Part model, mm, in its own coordinate system. Face numbers are marked on the shaded views. Give positions to 0.01 mm unless a question says otherwise; leave off trailing zeros. Order: outer loops, then holes, each group sorted by start corner. A loop starts at its lowest first (then second) coordinate and runs counter-clockwise, first axis right, second up. Notation, with made-up numbers: (69, -35.75) - (120, -35.75) arc R24 cw to (120, -15.75) - close; hole circle Ø3 at (67, 42.5). An arc over 180 degrees is marked (long way). One line per item, written item: value.
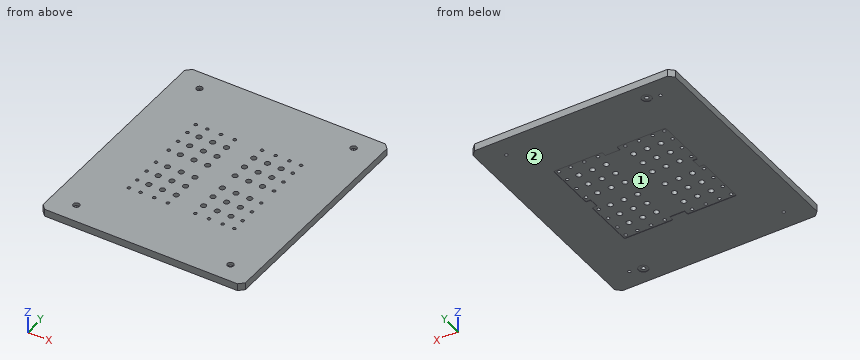
```python
from build123d import *

# Parameters (mm, degrees)
F0_W           = 210
F0_H           = 240
F1_DEPTH       = 7.5
F3_D           = 3.15
F3_CBORE_D     = 6.5
F3_CBORE_DEPTH = 3
F5_D           = 4.2
F5_DEPTH       = 5.5
F5_CBORE_D     = 10
F5_CBORE_DEPTH = 0.5
F5_TIP         = 1.2618073
F7_D           = 5.5
F9_D           = 3.3
F10_R          = 1.65
F10_R_2        = 2.75
F11_DEPTH      = 0.5
F12_SIZE       = 5
F13_R          = 1.5


with BuildPart() as f1:
    # F0 (on Top) → F1 (new body)
    with BuildSketch(Plane.XY):
        Rectangle(F0_W, F0_H)
    extrude(amount=F1_DEPTH)

    # F3 (through all)
    with Locations(Plane.XY.offset(7.5)):
        with Locations((-80, 100), (80, 100), (-80, -100), (80, -100)):
            CounterBoreHole(F3_D / 2, F3_CBORE_D / 2, F3_CBORE_DEPTH)

    # F5
    with Locations(Plane(origin=(0, 0, 0), x_dir=(1, 0, 0), z_dir=(0, 0, -1))):
        with Locations((-67.5, -103), (67.5, 103)):
            CounterBoreHole(F5_D / 2, F5_CBORE_D / 2, F5_CBORE_DEPTH, depth=F5_DEPTH)
            with Locations((0, 0, -(F5_DEPTH + F5_TIP / 2))):  # 118° drill point
                Cone(0, F5_D / 2, F5_TIP, mode=Mode.SUBTRACT)

    # F7 (through all)
    with Locations(Plane.XY.offset(7.5)):
        with Locations((-42.6, 40.75), (-28.4, 40.75), (-14.2, 40.75), (14.2, 40.75), (28.4, 40.75), (42.6, 40.75), (-42.6, 25.55), (-28.4, 25.55), (-14.2, 25.55), (14.2, 25.55), (28.4, 25.55), (42.6, 25.55), (42.6, 10.35), (28.4, 10.35), (14.2, 10.35), (-14.2, 10.35), (-28.4, 10.35), (-42.6, 10.35), (-42.6, -10.35), (-28.4, -10.35), (-14.2, -10.35), (14.2, -10.35), (28.4, -10.35), (42.6, -10.35), (42.6, -25.55), (28.4, -25.55), (14.2, -25.55), (-14.2, -25.55), (-28.4, -25.55), (-42.6, -25.55), (-42.6, -40.75), (-28.4, -40.75), (-14.2, -40.75), (14.2, -40.75), (28.4, -40.75), (42.6, -40.75)):
            Hole(F7_D / 2)

    # F9 (through all)
    with Locations(Plane.XY.offset(7.5)):
        with Locations((-54.65, 54.2), (-42.6, 54.2), (-28.4, 54.2), (-14.2, 54.2), (14.2, 54.2), (28.4, 54.2), (42.6, 54.2), (54.65, 54.2), (54.65, 40.75), (54.65, 25.55), (54.65, 10.35), (54.65, -10.35), (54.65, -25.55), (54.65, -40.75), (54.65, -54.2), (42.6, -54.2), (28.4, -54.2), (14.2, -54.2), (-14.2, -54.2), (-28.4, -54.2), (-42.6, -54.2), (-54.65, -54.2), (-54.65, -40.75), (-54.65, -25.55), (-54.65, -10.35), (-54.65, 10.35), (-54.65, 25.55), (-54.65, 40.75)):
            Hole(F9_D / 2)

    # F10 (on face) → F11 (cut)
    with BuildSketch(Plane(origin=(0, 0, 0), x_dir=(1, 0, 0), z_dir=(0, 0, -1))):
        with BuildLine():
            Line((7.5, -57.7), (56.625, -57.7))
            ThreePointArc((56.625, -57.7), (57.6856601718, -57.2606601718), (58.125, -56.2))
            Line((58.125, -56.2), (58.125, -5))
            Line((58.125, -5), (53.125, -5))
            Line((53.125, -5), (53.125, 5))
            Line((53.125, 5), (58.125, 5))
            Line((58.125, 5), (58.125, 56.2))
            ThreePointArc((58.125, 56.2), (57.6856601718, 57.2606601718), (56.625, 57.7))
            Line((56.625, 57.7), (7.5, 57.7))
            Line((7.5, 57.7), (7.5, 52.7))
            Line((7.5, 52.7), (-7.5, 52.7))
            Line((-7.5, 52.7), (-7.5, 57.7))
            Line((-7.5, 57.7), (-56.625, 57.7))
            ThreePointArc((-56.625, 57.7), (-57.6856601718, 57.2606601718), (-58.125, 56.2))
            Line((-58.125, 56.2), (-58.125, 5))
            Line((-58.125, 5), (-53.125, 5))
            Line((-53.125, 5), (-53.125, -5))
            Line((-53.125, -5), (-58.125, -5))
            Line((-58.125, -5), (-58.125, -56.2))
            ThreePointArc((-58.125, -56.2), (-57.6856601718, -57.2606601718), (-56.625, -57.7))
            Line((-56.625, -57.7), (-7.5, -57.7))
            Line((-7.5, -57.7), (-7.5, -52.7))
            Line((-7.5, -52.7), (7.5, -52.7))
            Line((7.5, -52.7), (7.5, -57.7))
        make_face()
        with Locations((-54.65, -54.2)):
            Circle(F10_R, mode=Mode.SUBTRACT)
        with Locations((-54.65, -40.75)):
            Circle(F10_R, mode=Mode.SUBTRACT)
        with Locations((-54.65, -25.55)):
            Circle(F10_R, mode=Mode.SUBTRACT)
        with Locations((-54.65, -10.35)):
            Circle(F10_R, mode=Mode.SUBTRACT)
        with Locations((-42.6, -54.2)):
            Circle(F10_R, mode=Mode.SUBTRACT)
        with Locations((-28.4, -54.2)):
            Circle(F10_R, mode=Mode.SUBTRACT)
        with Locations((-42.6, -40.75)):
            Circle(F10_R_2, mode=Mode.SUBTRACT)
        with Locations((-28.4, -40.75)):
            Circle(F10_R_2, mode=Mode.SUBTRACT)
        with Locations((-14.2, -54.2)):
            Circle(F10_R, mode=Mode.SUBTRACT)
        with Locations((-14.2, -40.75)):
            Circle(F10_R_2, mode=Mode.SUBTRACT)
        with Locations((-42.6, -25.55)):
            Circle(F10_R_2, mode=Mode.SUBTRACT)
        with Locations((-28.4, -25.55)):
            Circle(F10_R_2, mode=Mode.SUBTRACT)
        with Locations((-42.6, -10.35)):
            Circle(F10_R_2, mode=Mode.SUBTRACT)
        with Locations((-28.4, -10.35)):
            Circle(F10_R_2, mode=Mode.SUBTRACT)
        with Locations((-14.2, -25.55)):
            Circle(F10_R_2, mode=Mode.SUBTRACT)
        with Locations((-14.2, -10.35)):
            Circle(F10_R_2, mode=Mode.SUBTRACT)
        with Locations((14.2, -54.2)):
            Circle(F10_R, mode=Mode.SUBTRACT)
        with Locations((14.2, -40.75)):
            Circle(F10_R_2, mode=Mode.SUBTRACT)
        with Locations((28.4, -54.2)):
            Circle(F10_R, mode=Mode.SUBTRACT)
        with Locations((42.6, -54.2)):
            Circle(F10_R, mode=Mode.SUBTRACT)
        with Locations((28.4, -40.75)):
            Circle(F10_R_2, mode=Mode.SUBTRACT)
        with Locations((42.6, -40.75)):
            Circle(F10_R_2, mode=Mode.SUBTRACT)
        with Locations((14.2, -25.55)):
            Circle(F10_R_2, mode=Mode.SUBTRACT)
        with Locations((14.2, -10.35)):
            Circle(F10_R_2, mode=Mode.SUBTRACT)
        with Locations((28.4, -25.55)):
            Circle(F10_R_2, mode=Mode.SUBTRACT)
        with Locations((42.6, -25.55)):
            Circle(F10_R_2, mode=Mode.SUBTRACT)
        with Locations((28.4, -10.35)):
            Circle(F10_R_2, mode=Mode.SUBTRACT)
        with Locations((42.6, -10.35)):
            Circle(F10_R_2, mode=Mode.SUBTRACT)
        with Locations((54.65, -54.2)):
            Circle(F10_R, mode=Mode.SUBTRACT)
        with Locations((54.65, -40.75)):
            Circle(F10_R, mode=Mode.SUBTRACT)
        with Locations((54.65, -25.55)):
            Circle(F10_R, mode=Mode.SUBTRACT)
        with Locations((54.65, -10.35)):
            Circle(F10_R, mode=Mode.SUBTRACT)
        with Locations((-54.65, 10.35)):
            Circle(F10_R, mode=Mode.SUBTRACT)
        with Locations((-54.65, 25.55)):
            Circle(F10_R, mode=Mode.SUBTRACT)
        with Locations((-54.65, 40.75)):
            Circle(F10_R, mode=Mode.SUBTRACT)
        with Locations((-54.65, 54.2)):
            Circle(F10_R, mode=Mode.SUBTRACT)
        with Locations((-42.6, 10.35)):
            Circle(F10_R_2, mode=Mode.SUBTRACT)
        with Locations((-28.4, 10.35)):
            Circle(F10_R_2, mode=Mode.SUBTRACT)
        with Locations((-42.6, 25.55)):
            Circle(F10_R_2, mode=Mode.SUBTRACT)
        with Locations((-28.4, 25.55)):
            Circle(F10_R_2, mode=Mode.SUBTRACT)
        with Locations((-14.2, 10.35)):
            Circle(F10_R_2, mode=Mode.SUBTRACT)
        with Locations((-14.2, 25.55)):
            Circle(F10_R_2, mode=Mode.SUBTRACT)
        with Locations((-42.6, 40.75)):
            Circle(F10_R_2, mode=Mode.SUBTRACT)
        with Locations((-28.4, 40.75)):
            Circle(F10_R_2, mode=Mode.SUBTRACT)
        with Locations((-42.6, 54.2)):
            Circle(F10_R, mode=Mode.SUBTRACT)
        with Locations((-28.4, 54.2)):
            Circle(F10_R, mode=Mode.SUBTRACT)
        with Locations((-14.2, 40.75)):
            Circle(F10_R_2, mode=Mode.SUBTRACT)
        with Locations((-14.2, 54.2)):
            Circle(F10_R, mode=Mode.SUBTRACT)
        with Locations((14.2, 10.35)):
            Circle(F10_R_2, mode=Mode.SUBTRACT)
        with Locations((14.2, 25.55)):
            Circle(F10_R_2, mode=Mode.SUBTRACT)
        with Locations((28.4, 10.35)):
            Circle(F10_R_2, mode=Mode.SUBTRACT)
        with Locations((42.6, 10.35)):
            Circle(F10_R_2, mode=Mode.SUBTRACT)
        with Locations((28.4, 25.55)):
            Circle(F10_R_2, mode=Mode.SUBTRACT)
        with Locations((42.6, 25.55)):
            Circle(F10_R_2, mode=Mode.SUBTRACT)
        with Locations((14.2, 40.75)):
            Circle(F10_R_2, mode=Mode.SUBTRACT)
        with Locations((14.2, 54.2)):
            Circle(F10_R, mode=Mode.SUBTRACT)
        with Locations((28.4, 40.75)):
            Circle(F10_R_2, mode=Mode.SUBTRACT)
        with Locations((42.6, 40.75)):
            Circle(F10_R_2, mode=Mode.SUBTRACT)
        with Locations((28.4, 54.2)):
            Circle(F10_R, mode=Mode.SUBTRACT)
        with Locations((42.6, 54.2)):
            Circle(F10_R, mode=Mode.SUBTRACT)
        with Locations((54.65, 10.35)):
            Circle(F10_R, mode=Mode.SUBTRACT)
        with Locations((54.65, 25.55)):
            Circle(F10_R, mode=Mode.SUBTRACT)
        with Locations((54.65, 40.75)):
            Circle(F10_R, mode=Mode.SUBTRACT)
        with Locations((54.65, 54.2)):
            Circle(F10_R, mode=Mode.SUBTRACT)
    extrude(amount=-F11_DEPTH, mode=Mode.SUBTRACT)

    # F12
    f12_edges = [f1.edges().sort_by_distance(p)[0] for p in [
        (-105, 120, 3.75),
        (105, 120, 3.75),
        (-105, -120, 3.75),
        (105, -120, 3.75),
    ]]
    chamfer(f12_edges, length=F12_SIZE)

    # F13
    f13_edges = [f1.edges().sort_by_distance(p)[0] for p in [
        (7.5, 57.7, 0.25),
        (-7.5, 57.7, 0.25),
        (58.125, -5, 0.25),
        (58.125, 5, 0.25),
        (7.5, -57.7, 0.25),
        (-7.5, -57.7, 0.25),
        (-58.125, -5, 0.25),
        (-58.125, 5, 0.25),
    ]]
    fillet(f13_edges, radius=F13_R)


solid = f1.part
```
1) Two-plate mould, pull along X, no slides. Class the marked faces 1 and 2: pulls with the +X half, pulls with the -X half, needs draft (parallel to the pull), parting line crosses it, or undercut.
Answer:
face 1: undercut
face 2: needs draft
2) Drop flat-ended pins along their axis: P1, Ø5, axis at x = 80, y = -100, coming from the +Z side; P2, Ø6.5, axis at x = -42.6, y = -25.55, coming from the -Z side; P3, Ø2.5, axis at x = 67.5, y = -103, coming from the -Z side. Give the stop position or say it passes through.
Answer:
P1: stops at z = 4.5
P2: stops at z = 0.5
P3: stops at z = 6.01
3) Slice it at A-A on x = -0.5. Write the cut outline in (y, z).
Answer:
outline: (-120, 0) - (-52.7, 0) - (-52.7, 0.5) - (52.7, 0.5) - (52.7, 0) - (120, 0) - (120, 7.5) - (-120, 7.5) - close
4) Wall check: line 1 along Z through (x, y) = (-14.5, -15). Give the ranges that are in metal, low to high. Write a range as [from, to].
Answer:
line 1: z = [0.5, 7.5]
